Geometry check sheet. Reference: the model listing, model coordinates, mm. Coordinates: 2 decimals unless noted, no trailing zeros. Write each loop counter-clockwise with the first axis right and the second up, starting at its lowest first coordinate (ties: lowest second). Pieces come first, ordered by that corner, then holes. Notation, with made-up numbers: (24, 23.5) -> (76, 23.5) arc R15 cw to (76, 51.5) -> close; hole circle Ø4 at (-6, 20). An arc over 180 degrees is marked (long way). Answer in a Markdown table with one row per item. Add a question column.
Q1. Section check D-D, the plane y = 2. Record the boundary of the cut face in (x, z), and give its area (3 significant figures).
Q2. Gauge pin test, flat ends, axial feed: P1, Ø4, axis at y = 5, z = -8, coming from the -X side; P2, Ø2, axis at y = 5.5, z = 17.5, coming from the -X side; P3, Ø3, axis at y = 5.5, z = -2.5, coming from the -X side. Record the tip position at first contact, or that the pin passes through.
Q3. Section check C-C, the plane y = 6.75. Record the boundary of the cut face in (x, z).
Q4. Section check B-B, the plane x = 0. Record the boundary of the cut face in (y, z), and give its area (3 significant figures).
Q5. Section check A-A, the plane z = 0. Record the boundary of the cut face in (x, y), and give its area (3 significant figures).
Q6. Thickness scan on line 1 (Z direction, x = 0.5, y = 4.75) (3 decimals); line 2 (X direction, y = 4, z = -1); line 3 (Z direction, x = 21.5, y = 7). Record the ranges inside material, lowest first.
Q7. Release check for a two-part mould opening along Z. For faces 1 (the face through (-22.2, 4.2, 11.5)), 2 (the face through (0, 8.333, 0)) record: pulls with the +Z half, pulls with the -Z half, needs draft (parallel to the pull), parting line crosses it, or undercut.
```python
from build123d import *

# Parameters (mm, degrees)
SKETCH2_R           = 75
BOSS_EXTRUDE1_DEPTH = 25
FILLET1_R           = 10
SCALE1_SCALE        = 0.333333333


with BuildPart() as part:
    # Sketch2 → Boss-Extrude1 (new body)
    with BuildSketch(Plane(origin=(0, 0, 0), x_dir=(1, 0, 0), z_dir=(0, 1, 0))):
        with Locations(Location((0, 0, 0), (0, 0, 270))):
            Circle(SKETCH2_R)
    extrude(amount=BOSS_EXTRUDE1_DEPTH)

    # Fillet1
    fillet1_edges = [part.edges().sort_by_distance(p)[0] for p in [
        (0, 0, -75),
        (0, 25, -75),
    ]]
    fillet(fillet1_edges, radius=FILLET1_R)


with BuildPart() as part_1:
    # Scale1: scaled about (0, 0, 0)
    add(part.part.scale(SCALE1_SCALE))


solid = part_1.part
```
Calculated:
| question | item | result |
|---|---|---|
| 1 | outline | circle Ø49.44 at (0, 0) |
| 1 | area | 1,920 mm² |
| 2 | P1 | stops at x = -24.27 |
| 2 | P2 | stops at x = -18.75 |
| 2 | P3 | stops at x = -24.98 |
| 3 | outline | circle Ø49.01 at (0, 0) |
| 4 | outline | (0, -21.67) arc R3.33 ccw to (3.33, -25) -> (5, -25) arc R3.33 ccw to (8.33, -21.67) -> (8.33, 21.67) arc R3.33 ccw to (5, 25) -> (3.33, 25) arc R3.33 ccw to (0, 21.67) -> close |
| 4 | area | 407 mm² |
| 5 | outline | (-25, 3.33) arc R3.33 ccw to (-21.67, 0) -> (21.67, 0) arc R3.33 ccw to (25, 3.33) -> (25, 5) arc R3.33 ccw to (21.67, 8.33) -> (-21.67, 8.33) arc R3.33 ccw to (-25, 5) -> close |
| 5 | area | 407 mm² |
| 6 | line 1 | z = -24.995 to 24.995 |
| 6 | line 2 | x = -24.98 to 24.98 |
| 6 | line 3 | z = -11.4 to 11.4 |
| 7 | face 1 | parting line crosses it |
| 7 | face 2 | needs draft |
